Source: CAD feature listing. Evaluate the final solid. Frame: model axes, mm. Coordinates: 2 decimals unless noted, no trailing zeros. Order: outer loops, then holes, each group sorted by start corner. A loop starts at its lowest first (then second) coordinate and runs counter-clockwise, first axis right, second up. Notation, with made-up numbers: (18, -2) - (63, -2) arc R28 ccw to (63, 36) - close; hole circle Ø5 at (-5, -7). An arc over 180 degrees is marked (long way). One line per question, with ' | ' between items.
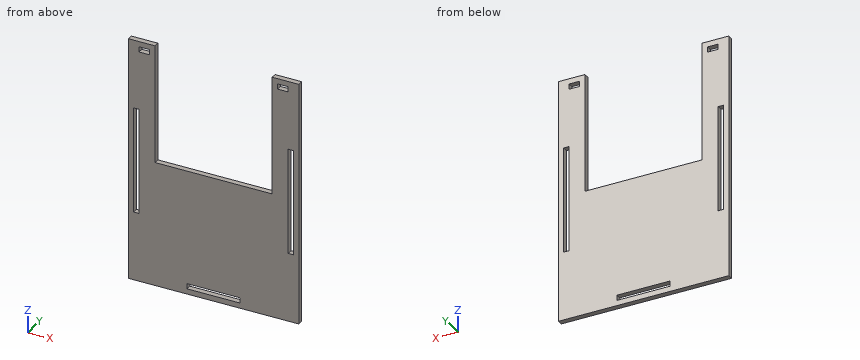
from build123d import *

# Parameters (mm, degrees)
SKETCH1_W           = 31.75
SKETCH1_H           = 3.175
SKETCH1_W_2         = 3.175
SKETCH1_H_2         = 63.5
SKETCH1_W_3         = 6.35
BOSS_EXTRUDE1_DEPTH = 3.175


with BuildPart() as part:
    # Sketch1 → Boss-Extrude1 (new body)
    with BuildSketch(Plane(origin=(0, 0, 0), x_dir=(1, 0, 0), z_dir=(0, 1, 0))):
        Polygon((-50.8, 73.025), (50.8, 73.025), (50.8, -73.025), (34.925, -73.025), (34.925, -1.905), (-34.925, -1.905), (-34.925, -73.025), (-50.8, -73.025), align=None)
        with Locations((0, 68.2625)):
            Rectangle(SKETCH1_W, SKETCH1_H, mode=Mode.SUBTRACT)
        with Locations((-46.0375, 0)):
            Rectangle(SKETCH1_W_2, SKETCH1_H_2, mode=Mode.SUBTRACT)
        with Locations((46.0375, 0)):
            Rectangle(SKETCH1_W_2, SKETCH1_H_2, mode=Mode.SUBTRACT)
        with Locations((-41.275, -68.2625)):
            Rectangle(SKETCH1_W_3, SKETCH1_H, mode=Mode.SUBTRACT)
        with Locations((41.275, -68.2625)):
            Rectangle(SKETCH1_W_3, SKETCH1_H, mode=Mode.SUBTRACT)
    extrude(amount=BOSS_EXTRUDE1_DEPTH)


solid = part.part
(1) Cut plane A-A (x = 6). Return the cut outline in (y, z) (3 decimals), and give its area (3 significant figures).
Taken from the geometry:
outline: (0, -73.025) - (3.175, -73.025) - (3.175, -69.85) - (0, -69.85) - close; (0, -66.675) - (3.175, -66.675) - (3.175, 1.905) - (0, 1.905) - close | area: 228 mm²
(2) Cut plane D-D (z = -23.5). Return the cut outline in (x, y) (3 decimals), and give its area (3 significant figures).
Taken from the geometry:
outline: (-50.8, 0) - (-47.625, 0) - (-47.625, 3.175) - (-50.8, 3.175) - close; (-44.45, 0) - (44.45, 0) - (44.45, 3.175) - (-44.45, 3.175) - close; (47.625, 0) - (50.8, 0) - (50.8, 3.175) - (47.625, 3.175) - close | area: 302 mm²
(3) Cut plane B-B (z = 37). Return the cut outline in (x, y) (3 decimals).
Taken from the geometry:
outline: (-50.8, 0) - (-34.925, 0) - (-34.925, 3.175) - (-50.8, 3.175) - close; (34.925, 0) - (50.8, 0) - (50.8, 3.175) - (34.925, 3.175) - close
(4) Material intervals for L1, parallel to X at y = 1.3, z = 28.5 (3 decimals); L2, parallel to Z at x = 14, y = 1.75 (3 decimals); L3, parallel to X at y = 1.25, z = -6.5 (3 decimals), sorted ascending. Write a range as from..to.
Taken from the geometry:
L1: x = -50.8..-47.625, -44.45..-34.925, 34.925..44.45, 47.625..50.8 | L2: z = -73.025..-69.85, -66.675..1.905 | L3: x = -50.8..-47.625, -44.45..44.45, 47.625..50.8
(5) Pin query (flat end, axial travel): P1, Ø1.6, axis at x = -2, y = 1.5, coming from the +Z side (3 decimals). Return the tip coordinate at first contact, or that it passes through.
Taken from the geometry:
P1: stops at z = 1.905
(6) Cut plane C-C (y = 2.6). Return the cut outline in (x, z) (3 decimals), and give its area (3 significant figures).
Taken from the geometry:
outline: (-50.8, -73.025) - (50.8, -73.025) - (50.8, 73.025) - (34.925, 73.025) - (34.925, 1.905) - (-34.925, 1.905) - (-34.925, 73.025) - (-50.8, 73.025) - close; hole (-47.625, -31.75) - (-44.45, -31.75) - (-44.45, 31.75) - (-47.625, 31.75) - close; hole (-44.45, 66.675) - (-38.1, 66.675) - (-38.1, 69.85) - (-44.45, 69.85) - close; hole (-15.875, -69.85) - (15.875, -69.85) - (15.875, -66.675) - (-15.875, -66.675) - close; hole (38.1, 66.675) - (44.45, 66.675) - (44.45, 69.85) - (38.1, 69.85) - close; hole (44.45, -31.75) - (47.625, -31.75) - (47.625, 31.75) - (44.45, 31.75) - close | area: 9,330 mm²
